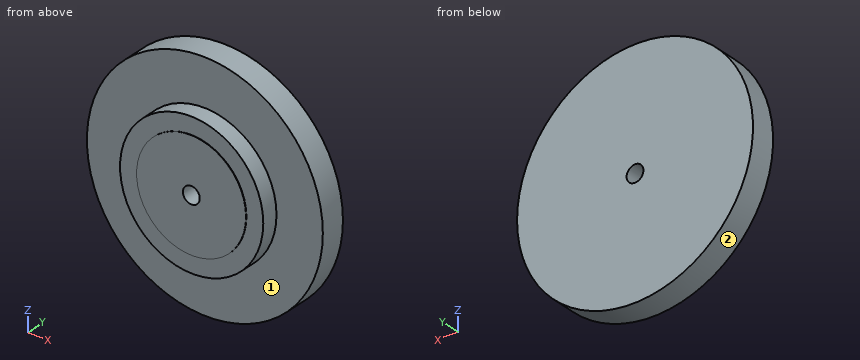
```python
from build123d import *

# Parameters (mm, degrees)
F0_R     = 20.6375
F0_R_2   = 3.175
F1_DEPTH = 16.1544
F0_R_3   = 26.9875
F2_DEPTH = 16.002
F0_R_4   = 44.45
F3_DEPTH = 9.652


with BuildPart() as f1:
    # F0 (on Front) → F1 (new body)
    with BuildSketch(Plane.XZ):
        Circle(F0_R)
        Circle(F0_R_2, mode=Mode.SUBTRACT)
    extrude(amount=F1_DEPTH)

    # F0 (on Front) → F2 (join)
    with BuildSketch(Plane.XZ):
        Circle(F0_R_3)
        Circle(F0_R, mode=Mode.SUBTRACT)
    extrude(amount=F2_DEPTH)

    # F0 (on Front) → F3 (join)
    with BuildSketch(Plane.XZ):
        Circle(F0_R_4)
        Circle(F0_R_3, mode=Mode.SUBTRACT)
    extrude(amount=F3_DEPTH)


solid = f1.part
```
Could you check a few things on this model? Use its own coordinates, in mm. Face numbers are marked on the shaded views. A direction names the side the tool comes from. Give positions to 0.01 mm unless a question says otherwise; leave off trailing zeros. Write each loop counter-clockwise with the first axis right and the second up, starting at its lowest first coordinate (ties: lowest second). Pieces come first, ordered by that corner, then holes. Notation, with made-up numbers: (79.25, 11.5) - (112.25, 11.5) arc R19 ccw to (112.25, 20.5) - close; hole circle Ø2 at (-23.5, 71.5). An arc over 180 degrees is marked (long way). One line per item, written item: value. Start each with the question number.
Item 1: Imagine slicing it at D-D, the plane z = -19. List the corners of the cut face in (x, y) for me, and give its area (3 significant figures).
Item 2: Which directions (+Z, -Z, +X, -X, +Y, -Y) give clear straight access to the entire face, cutting with the end or side of a thin tool? Please do the marked faces 1 and 2.
Item 3: Please list where these lines run through material, in increasing order: line 1 (Z direction, x = 0, y = -4.5) (3 decimals); line 2 (Z direction, x = 0, y = -11.25) (1 decimal); line 3 (Y direction, x = 27, z = -4). Write a range as from..to.
Item 4: Imagine slicing it at C-C, the plane y = -6.25. List the corners of the cut face in (x, z) for me (3 decimals).
Item 5: I'm going to push flat-ended pins straight in: pin 1 (10 mm diameter, centred on x = -1, z = 14, fed in from +Y); pin 2 (5 mm diameter, centred on x = 4.5, y = -5.5, fed in from +Z) (3 decimals); pin 3 (1 mm diameter, centred on x = -26.5, y = -5.5, fed in from +Z); pin 4 (3 mm diameter, centred on x = -13.5, z = -23.5, fed in from -Y). Where does each tip first touch, or does it pass through?
Geometry says:
1. outline: (-40.18, -9.65) - (-19.17, -9.65) - (-19.17, -16) - (-8.06, -16) - (-8.06, -16.15) - (8.06, -16.15) - (8.06, -16) - (19.17, -16) - (19.17, -9.65) - (40.18, -9.65) - (40.18, 0) - (-40.18, 0) - close
1. area: 1,020 mm^2
2. face 1: -Y
2. face 2: +Y, -Y
3. line 1: -44.45..-3.175, 3.175..44.45
3. line 2: -27..-3.2, 3.2..27
3. line 3: -9.65..0
4. outline: circle Ø88.9 at (0, 0); hole circle Ø6.35 at (0, 0)
5. pin 1: y = 0
5. pin 2: z = 44.405
5. pin 3: z = 36.05
5. pin 4: y = -16
